from build123d import *

# Parameters (mm, degrees)
F0_W     = 23
F0_H     = 12.4
F0_R     = 1.5
F1_DEPTH = 5.4
F2_SIZE  = 1
F3_R     = 2.9
F3_R_2   = 1.5
F4_DEPTH = 5
F5_R     = 3.5
F5_R_2   = 3
F6_DEPTH = 2.5
F7_DEPTH = 3.5
F8_R     = 1.5
F9_DEPTH = 10


with BuildPart() as f1:
    # F0 (on Top) → F1 (new body)
    with BuildSketch(Plane.XY):
        with Locations((11.5, 6.2)):
            Rectangle(F0_W, F0_H)
        with Locations((19, 6.2)):
            Circle(F0_R, mode=Mode.SUBTRACT)
    extrude(amount=F1_DEPTH)

    # F2
    f2_edges = [f1.edges().sort_by_distance(p)[0] for p in [
        (11.5, 0, 0),
        (11.5, 12.4, 0),
    ]]
    chamfer(f2_edges, length=F2_SIZE)

    # F3 (on face) → F4 (join)
    with BuildSketch(Plane.XY.offset(5.4)):
        with Locations((19, 6.2)):
            Circle(F3_R)
        with Locations((19, 6.2)):
            Circle(F3_R_2, mode=Mode.SUBTRACT)
    extrude(amount=F4_DEPTH)

    # F5 (on face) → F6 (join)
    with BuildSketch(Plane(origin=(0, 0, 0), x_dir=(1, 0, 0), z_dir=(0, 0, -1))):
        with Locations((19, -6.2)):
            Circle(F5_R)
        with Locations((19, -6.2)):
            Circle(F5_R_2, mode=Mode.SUBTRACT)
    extrude(amount=F6_DEPTH)

    # F7 (cut): a face of the model
    f7_faces = [f1.faces().sort_by_distance(p)[0] for p in [
        (16.0848528137, 6.2, 0),
    ]]
    extrude(f7_faces, amount=-F7_DEPTH, mode=Mode.SUBTRACT)

    # F8 (on face) → F9 (join)
    with BuildSketch(Plane.XY.offset(5.4)):
        with Locations((12, 6.2)):
            Circle(F8_R)
    extrude(amount=F9_DEPTH)


solid = f1.part
Can you work these out from the model? Positions are in its coordinate system, mm. A direction names the side the tool comes from. Give positions to 0.01 mm unless a question says otherwise; leave off trailing zeros. Order: outer loops, then holes, each group sorted by start corner. A loop starts at its lowest first (then second) coordinate and runs counter-clockwise, first axis right, second up. Notation, with made-up numbers: M -2.5,19.25 L 11.5,19.25 A31 ccw 11.5,48.25 Z; hole C 57.5,12.5 d4. An arc over 180 degrees is marked long. One line per question, with ' | ' between items.
Item 1: We'd pull the mould along X, two halves only. Please class faces 4 (the face through (20, 8, 3.5)), 5 (the face through (23, 6, 3)), 6 (the face through (11, 12.4, 3)), 7 (the face through (17.8, 5.3, 6.9)): released by +X, released by -X, zero draft, split by the parting line, or undercut.
Answer block:
face 4: undercut | face 5: released by +X | face 6: zero draft | face 7: undercut
Item 2: I'm going to push flat-ended pins straight in: pin 1 Ø3 at (x, y) = (8, 8.5) entering from -Z; pin 2 Ø7 at (x, y) = (19, 6.2) entering from -Z; pin 3 Ø1 at (x, y) = (16, 9) entering from +Z; pin 4 Ø2.5 at (x, y) = (19, 6.2) entering from -Z. Where does each tip first touch, or does it pass through?
Answer block:
pin 1: stops at z = 0 | pin 2: stops at z = -2.5 | pin 3: stops at z = 5.4 | pin 4: passes through
Item 3: Please list where these lines run through material, in increasing order: L1, parallel to X at y = 6.2, z = 2.3; L2, parallel to Y at x = 19, z = 6; L3, parallel to Y at x = 19, z = 1.15.
Answer block:
L1: x = 0 to 16, 22 to 23 | L2: y = 3.3 to 4.7, 7.7 to 9.1 | L3: y = 0 to 3.2, 9.2 to 12.4
Item 4: Suppose I cut it at B-B, the plane y = 6.2. Write out the boundary of the cut face in (x, z).
Answer block:
outline: M 0,0 L 15.5,0 L 15.5,-2.5 L 16,-2.5 L 16,3.5 L 17.5,3.5 L 17.5,10.4 L 16.1,10.4 L 16.1,5.4 L 13.5,5.4 L 13.5,15.4 L 10.5,15.4 L 10.5,5.4 L 0,5.4 Z; M 20.5,3.5 L 22,3.5 L 22,-2.5 L 22.5,-2.5 L 22.5,0 L 23,0 L 23,5.4 L 21.9,5.4 L 21.9,10.4 L 20.5,10.4 Z
Item 5: Suppose I cut it at D-D, the plane x = 12. Write out the boundary of the cut face in (y, z), then the cut area to 3 significant figures.
Answer block:
outline: M 0,1 L 1,0 L 11.4,0 L 12.4,1 L 12.4,5.4 L 7.7,5.4 L 7.7,15.4 L 4.7,15.4 L 4.7,5.4 L 0,5.4 Z | area: 96.0 mm2
Item 6: For faces 1 (the face through (20.2, 5, 10.4)), 2 (the face through (22, 8, -1)), 3 (the face through (11.675, 4.736, 10.33)), which set-ups out of +Z, -Z, +X, -X, +Y, -Y let a thin tool reach every point of the face, with its end or its side?
Answer block:
face 1: +Z, +X, +Y, -Y | face 2: -Z | face 3: +Z
Item 7: Suppose I cut it at C-C, the plane z = 7.75. Write out the boundary of the cut face in (x, y), then the cut area to 3 significant figures.
Answer block:
outline: C 12,6.2 d3; C 19,6.2 d5.8; hole C 19,6.2 d3 | area: 26.4 mm2
Item 8: Suppose I cut it at A-A, the plane x = 19. Write out the boundary of the cut face in (y, z), then the cut area to 3 significant figures.
Answer block:
outline: M 0,1 L 1,0 L 2.7,0 L 2.7,-2.5 L 3.2,-2.5 L 3.2,3.5 L 4.7,3.5 L 4.7,10.4 L 3.3,10.4 L 3.3,5.4 L 0,5.4 Z; M 7.7,3.5 L 9.2,3.5 L 9.2,-2.5 L 9.7,-2.5 L 9.7,0 L 11.4,0 L 12.4,1 L 12.4,5.4 L 9.1,5.4 L 9.1,10.4 L 7.7,10.4 Z | area: 55.8 mm2
